Verification items for the finished model (mm, model axes). A direction names the side the tool comes from. Round coordinates to 2 decimals unless told otherwise and drop trailing zeros. Loops run counter-clockwise (first coordinate to the right, second up) from the corner with the lowest first, then second, coordinate; pieces in that order, holes last. Notation, with made-up numbers: M 37,-7.5 L 73,-7.5 A12 ccw 73,10.5 Z; hole C -31,45 d8. An arc over 180 degrees is marked long. One line per item, written item: value.
from build123d import *

# Parameters (mm, degrees)
SKETCH1_R           = 20
SKETCH1_R_2         = 11.35
SKETCH1_R_3         = 1.9
BOSS_EXTRUDE1_DEPTH = 5
CHAMFER1_SIZE       = 3
CHAMFER1_SIZE2      = 0.803847577
BOSS_EXTRUDE2_START = -2
SKETCH2_R           = 11.35
SKETCH2_R_2         = 9.85
BOSS_EXTRUDE2_DEPTH = 2
CHAMFER2_SIZE       = 1.5


with BuildPart() as part:
    # Sketch1 → Boss-Extrude1 (new body)
    with BuildSketch(Plane(origin=(0, 0, 0), x_dir=(1, 0, 0), z_dir=(0, 1, 0))):
        with Locations(Location((0, 0, 0), (0, 0, 270))):
            Circle(SKETCH1_R)
        with Locations(Location((0, 0, 0), (0, 0, 270))):
            Circle(SKETCH1_R_2, mode=Mode.SUBTRACT)
        with Locations(Location((0, 16, 0), (0, 0, 270))):
            Circle(SKETCH1_R_3, mode=Mode.SUBTRACT)
        with Locations(Location((16, 0, 0), (0, 0, 270))):
            Circle(SKETCH1_R_3, mode=Mode.SUBTRACT)
        with Locations(Location((0, -16, 0), (0, 0, 270))):
            Circle(SKETCH1_R_3, mode=Mode.SUBTRACT)
        with Locations(Location((-16, 0, 0), (0, 0, 270))):
            Circle(SKETCH1_R_3, mode=Mode.SUBTRACT)
    extrude(amount=BOSS_EXTRUDE1_DEPTH)

    # Chamfer1
    chamfer1_edges = [part.edges().sort_by_distance(p)[0] for p in [
        (0, 5, -20),
    ]]
    chamfer1_side = [part.faces().sort_by_distance(p)[0] for p in [
        (0, 2.5, -20),
    ]]
    chamfer(chamfer1_edges, length=CHAMFER1_SIZE, length2=CHAMFER1_SIZE2, reference=chamfer1_side[0])

    # Sketch2 → Boss-Extrude2 (add)
    with BuildSketch(Plane(origin=(0, 5, 0), x_dir=(1, 0, 0), z_dir=(0, 1, 0)).offset(BOSS_EXTRUDE2_START)):
        with Locations(Location((0, 0, 0), (0, 0, 270))):
            Circle(SKETCH2_R)
        with Locations(Location((0, 0, 0), (0, 0, 270))):
            Circle(SKETCH2_R_2, mode=Mode.SUBTRACT)
    extrude(amount=BOSS_EXTRUDE2_DEPTH)

    # Chamfer2
    chamfer2_edges = [part.edges().sort_by_distance(p)[0] for p in [
        (0, 3, -9.85),
    ]]
    chamfer(chamfer2_edges, length=CHAMFER2_SIZE - 0.0001)  # a hair under: the kernel refuses the full size


solid = part.part
(1) Sectioned sample at A-A on z = 0. Count the separate pieces of the cut face and the enclosed holes in it, and give its area (3 significant figures).
Completed:
separate pieces: 4
enclosed holes: 0
area: 49.8 mm^2
(2) Thickness scan on L1, parallel to X at y = 4.75, z = 0; L2, parallel to X at y = 4.5, z = -0.5; L3, parallel to Z at x = -8.5, y = 2.2. Record the ranges inside material, lowest first. Write a range as from..to.
Completed:
L1: x = -19.26..-17.9, -14.1..-9.85, 9.85..14.1, 17.9..19.26
L2: x = -19.32..-17.83, -14.17..-9.84, 9.84..14.17, 17.83..19.32
L3: z = -18.04..-7.52, 7.52..18.04
(3) Sectioned sample at B-B on y = 0.65. Enter the section's corners in (x, z), and give its area (3 significant figures).
Completed:
outline: C 0,0 d40; hole C -16,0 d3.8; hole C 0,0 d22.7; hole C 0,-16 d3.8; hole C 0,16 d3.8; hole C 16,0 d3.8
area: 807 mm^2
(4) Mould release check, pull along X, two halves, no side actions. Record for faces 3 (the face through (0.08, 2.46, 14.1)), 4 (the face through (19.071, 4.854, -2.504)), 5 (the face through (-9, 0, 9)), 6 (the face through (0.08, 2.46, -17.9)): +X half, -X half, draft (parallel to the pull), parting line (faces both ways), or undercut.
Completed:
face 3: undercut
face 4: parting line
face 5: draft
face 6: undercut
(5) Depth check by flat-ended pin: pin 1 Ø20.5 at (x, z) = (0, 0) entering from -Y; pin 2 Ø3 at (x, y) = (-0.5, 4.5) entering from +Z; pin 3 Ø2 at (x, y) = (-6.5, 0.5) entering from -Z. Enter the tip coordinate at first touch or a pass-through.
Completed:
pin 1: stops at y = 4.1
pin 2: stops at z = 19.73
pin 3: stops at z = -19.23
(6) Tool access check on faces 1 (the face through (-9.616, 4.746, -2.135)), 2 (the face through (-6.906, 1.479, -9.007)). Record the directions out of +Z, -Z, +X, -X, +Y, -Y that give a thin tool (end or side, any length) a straight path to the whole face; none if there is none.
Completed:
face 1: +Y, -Y
face 2: -Y
